Geometry check sheet. Reference: the model listing, model coordinates, mm. A direction names the side the tool comes from. Give positions to 0.01 mm unless a question says otherwise; leave off trailing zeros. Loops run counter-clockwise (first coordinate to the right, second up) from the corner with the lowest first, then second, coordinate; pieces in that order, holes last. Notation, with made-up numbers: (-37.5, 18.25) -> (4.5, 18.25) arc R21 ccw to (4.5, 47.25) -> close; hole circle Ø1 at (72.5, 41). An arc over 180 degrees is marked (long way). Write each question's results on one line, items separated by ' | '. Start each with the question number.
1) Scan lines: line 1 (Y direction, x = 12.75, z = 338.7); line 2 (Y direction, x = 9, z = 338.2). Record each from-to range of solid material in increasing order. Write a range as from..to.
2) Set-up check for faces 4 (the face through (-4.22, 13.38, 338.76)), 5 (the face through (-9.007, -10.723, 338.76)), 6 (the face through (-1.22, -13.98, 338.76)), 7 (the face through (6.48, 12.45, 338.76)): record each of +Z, -Z, +X, -X, +Y, -Y from which the full face is reachable in a straight line by a thin tool's end or side.
3) Sectioned sample at B-B on x = 10.5. Record the cut outline in (y, z).
4) Sectioned sample at A-A on y = 6.25. Record the cut outline in (x, z), then the cut area to 3 significant figures.
5) Draft check along Y on faces 1 (the face through (6.46, -12.424, 338.76)), 2 (the face through (13.98, -1.22, 338.76)), 3 (the face through (8.35, 12.46, 338.74)). Enter one of: pulls with the +Y half, pulls with the -Y half, needs draft (parallel to the pull), parting line crosses it, or undercut.
```python
from build123d import *

# Parameters (mm, degrees)
SKETCH012_R        = 15
PAD010_DEPTH       = 1.5
POCKET_DEPTH       = 84.90683
POCKET_DEPTH_BACK  = 86.40683
POLARPATTERN_COUNT = 16


with BuildPart() as part:
    # Sketch012 → Pad010 (new body)
    with BuildSketch(Plane.XY):
        Circle(SKETCH012_R)
    extrude(amount=PAD010_DEPTH)

    # Sketch013 → Pocket (cut, two sides)
    with BuildSketch(Plane.XY) as pocket_sk:
        with BuildLine():
            Line((-2, 17), (2, 17))
            Line((2, 17), (0.968311, 13))
            ThreePointArc((-0.968311, 13), (0, 12.249749), (0.968311, 13))
            Line((-0.968311, 13), (-2, 17))
        make_face()
    pocket = extrude(amount=-POCKET_DEPTH, mode=Mode.SUBTRACT) + extrude(pocket_sk.sketch, amount=POCKET_DEPTH_BACK, mode=Mode.SUBTRACT)

    # PolarPattern: Pocket ×16 about axis
    polarpattern_axis = Axis((0, 0, 0), (0, 0, 1))
    for i in range(1, POLARPATTERN_COUNT):
        add(pocket.rotate(polarpattern_axis, i * 360 / POLARPATTERN_COUNT), mode=Mode.SUBTRACT)


with BuildPart() as part_1:
    # Body011 placement: moved
    add(part.part.moved(Location((0, 0, 338))))


solid = part_1.part
```
Result:
1) line 1: -7.9..-6.7, -4.13..-0.87, 0.87..4.13, 6.7..7.9 | line 2: -12..-10.71, -8.44..8.44, 10.71..12
2) face 4: +Z, -Z | face 5: +Z, -Z, -X | face 6: +Z, -Z, -Y | face 7: +Z, -Z, +Y
3) outline: (-8.88, 338) -> (8.88, 338) -> (8.88, 339.5) -> (-8.88, 339.5) -> close
4) outline: (-12.15, 338) -> (12.15, 338) -> (12.15, 339.5) -> (-12.15, 339.5) -> close | area: 36.4 mm^2
5) face 1: pulls with the -Y half | face 2: undercut | face 3: pulls with the +Y half
